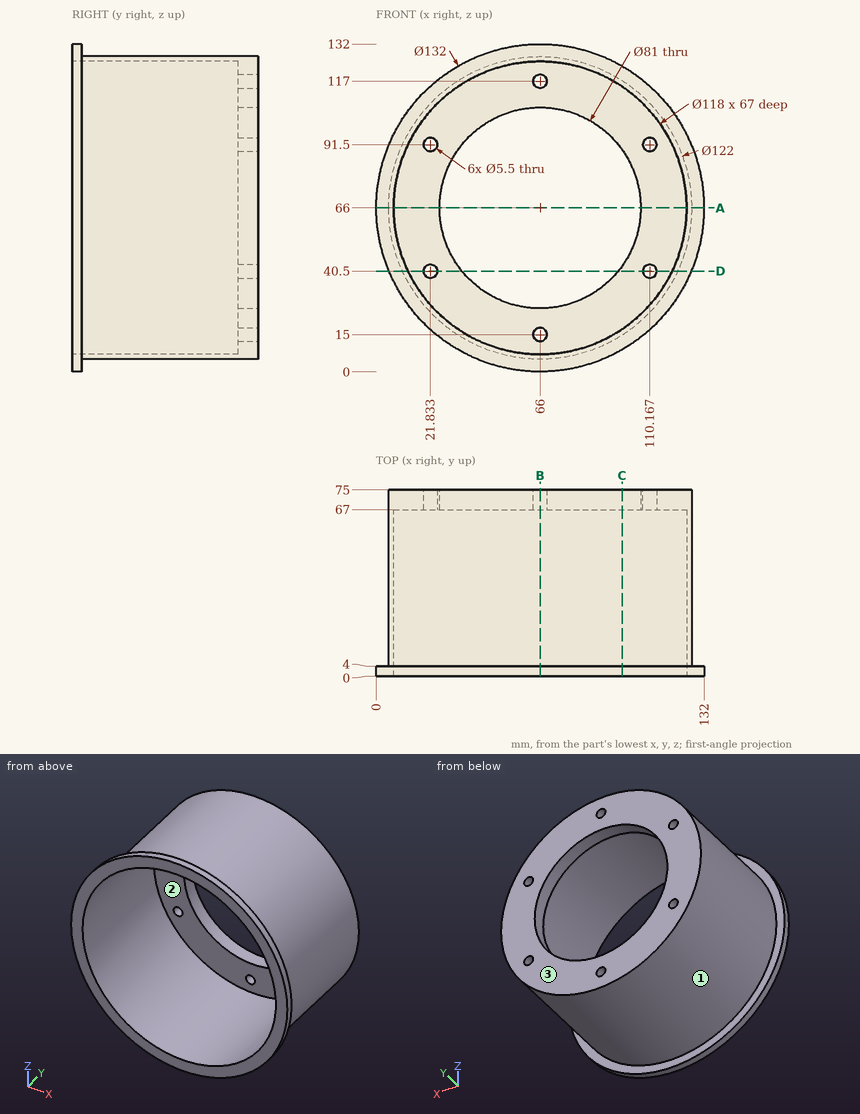
Here's the drawing with two shaded views (mm, measured from the low corner). I have some questions. A direction names the side the tool comes from. Round coordinates to 2 decimals unless told otherwise and drop trailing zeros. Loops run counter-clockwise (first coordinate to the right, second up) from the corner with the lowest first, then second, coordinate; pieces in that order, holes last.
Item 1: Suppose I cut it at C-C, the plane x = 99. Write out the boundary of the cut face in (y, z), then the cut area to 3 significant figures.
Item 2: Please list where these lines run through material, in increasing order: L1, parallel to X at y = 69.5, z = 91.5 (1 decimal); L2, parallel to Z at x = 66, y = 41.5; L3, parallel to Y at x = 15, z = 73.
Item 3: Suppose I cut it at B-B, the plane x = 66. Write out the boundary of the cut face in (y, z).
Item 4: Suppose I cut it at D-D, the plane z = 40.5. Write out the boundary of the cut face in (x, y) (1 decimal).
Item 5: Suppose I cut it at A-A, the plane z = 66. Write out the boundary of the cut face in (x, y).
Item 6: Which directions (+Z, -Z, +X, -X, +Y, -Y) give clear straight access to the entire face, cutting with the end or side of a thin tool? Please do the marked faces 1, 2 and 3.
Item 7: Will these pins go through, and if not, where does the flat tip stop? pin 1 Ø3 at (x, y) = (32, 18) entering from +Z; pin 2 Ø1 at (x, y) = (97.5, 60.5) entering from -Z (1 decimal); pin 3 Ø6.5 at (x, z) = (66, 15) entering from -Y.
Reported:
1. outline: (0, 8.84) - (4, 8.84) - (4, 14.7) - (75, 14.7) - (75, 42.52) - (67, 42.52) - (67, 17.09) - (0, 17.09) - close; (0, 114.91) - (67, 114.91) - (67, 89.48) - (75, 89.48) - (75, 117.3) - (4, 117.3) - (4, 123.16) - (0, 123.16) - close
1. area: 813 mm2
2. L1: x = 10.6 to 19.1, 24.6 to 34.5, 97.5 to 107.4, 112.9 to 121.4
2. L2: z = 5 to 7, 125 to 127
2. L3: y = 67 to 75
3. outline: (0, 0) - (4, 0) - (4, 5) - (75, 5) - (75, 12.25) - (67, 12.25) - (67, 7) - (0, 7) - close; (0, 125) - (67, 125) - (67, 119.75) - (75, 119.75) - (75, 127) - (4, 127) - (4, 132) - (0, 132) - close; (67, 17.75) - (75, 17.75) - (75, 25.5) - (67, 25.5) - close; (67, 106.5) - (75, 106.5) - (75, 114.25) - (67, 114.25) - close
4. outline: (5.1, 0) - (12.8, 0) - (12.8, 67) - (19.1, 67) - (19.1, 75) - (10.6, 75) - (10.6, 4) - (5.1, 4) - close; (24.6, 67) - (34.5, 67) - (34.5, 75) - (24.6, 75) - close; (97.5, 67) - (107.4, 67) - (107.4, 75) - (97.5, 75) - close; (112.9, 67) - (119.2, 67) - (119.2, 0) - (126.9, 0) - (126.9, 4) - (121.4, 4) - (121.4, 75) - (112.9, 75) - close
5. outline: (0, 0) - (7, 0) - (7, 67) - (25.5, 67) - (25.5, 75) - (5, 75) - (5, 4) - (0, 4) - close; (106.5, 67) - (125, 67) - (125, 0) - (132, 0) - (132, 4) - (127, 4) - (127, 75) - (106.5, 75) - close
6. face 1: +Y
6. face 2: -Y
6. face 3: +Z, -Z, +X, -X, +Y
7. pin 1: stops at z = 117.62
7. pin 2: stops at z = 13.5
7. pin 3: stops at y = 67
